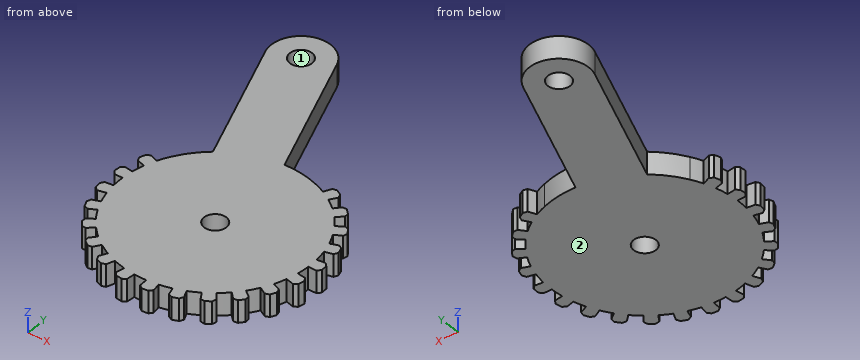
from build123d import *

# Parameters (mm, degrees)
SKETCH1_R           = 1.5
BOSS_EXTRUDE2_DEPTH = 3


with BuildPart() as part:
    # Sketch1 → Boss-Extrude2 (new body)
    with BuildSketch(Plane.XY):
        with BuildLine():
            Line((-15.222508379, 27.299729644), (-8.208462227, 9.756210733))
            ThreePointArc((-8.208462227, 9.756210733), (-9.850646229, 8.094891529), (-11.162172719, 6.161850387))
            ThreePointArc((-11.162172719, 6.161850387), (-11.536544919, 5.428685967), (-11.862823992, 4.672890641))
            Line((-11.862823992, 4.672890641), (-12.909543756, 5.085204521))
            Line((-12.909543756, 5.085204521), (-13.417390562, 4.799596912))
            Line((-13.417390562, 4.799596912), (-13.676029266, 4.003588828))
            Line((-13.676029266, 4.003588828), (-13.43304851, 3.474022556))
            Line((-13.43304851, 3.474022556), (-12.343882415, 3.192345052))
            ThreePointArc((-12.343882415, 3.192345052), (-12.524162447, 2.389111761), (-12.652232208, 1.575918828))
            Line((-12.652232208, 1.575918828), (-13.768605638, 1.71497049))
            Line((-13.768605638, 1.71497049), (-14.189469779, 1.312039404))
            Line((-14.189469779, 1.312039404), (-14.242023712, 0.476718548))
            Line((-14.242023712, 0.476718548), (-13.874978867, 0.024216431))
            Line((-13.874978867, 0.024216431), (-12.749980581, 0.022252937))
            ThreePointArc((-12.749980581, 0.022252937), (-12.724840787, -0.800579124), (-12.646654143, -1.62007376))
            Line((-12.646654143, -1.62007376), (-13.762535391, -1.763021444))
            Line((-13.762535391, -1.763021444), (-14.069972424, -2.257958364))
            Line((-14.069972424, -2.257958364), (-13.91313943, -3.080105712))
            Line((-13.91313943, -3.080105712), (-13.445093273, -3.427111302))
            Line((-13.445093273, -3.427111302), (-12.354950575, -3.149237412))
            ThreePointArc((-12.354950575, -3.149237412), (-12.125970583, -3.939966678), (-11.846440287, -4.714271155))
            Line((-11.846440287, -4.714271155), (-12.89171443, -5.130236257))
            Line((-12.89171443, -5.130236257), (-13.066406957, -5.686080305))
            Line((-13.066406957, -5.686080305), (-12.710041429, -6.443395602))
            Line((-12.710041429, -6.443395602), (-12.170403021, -6.663101027))
            Line((-12.170403021, -6.663101027), (-11.183613587, -6.122849592))
            ThreePointArc((-11.183613587, -6.122849592), (-10.76518105, -6.831791636), (-10.30187102, -7.512253556))
            Line((-10.30187102, -7.512253556), (-11.210859639, -8.175099458))
            Line((-11.210859639, -8.175099458), (-11.241831085, -8.756924908))
            Line((-11.241831085, -8.756924908), (-10.70832478, -9.401823249))
            Line((-10.70832478, -9.401823249), (-10.131001588, -9.48042361))
            Line((-10.131001588, -9.48042361), (-9.309569027, -8.711740614))
            ThreePointArc((-9.309569027, -8.711740614), (-8.727975601, -9.29435), (-8.109997309, -9.838213438))
            Line((-8.109997309, -9.838213438), (-8.825585306, -10.706291095))
            Line((-8.825585306, -10.706291095), (-8.710889622, -11.277539713))
            Line((-8.710889622, -11.277539713), (-8.033764703, -11.769499764))
            Line((-8.033764703, -11.769499764), (-7.455032066, -11.702056311))
            Line((-7.455032066, -11.702056311), (-6.850570006, -10.753240934))
            ThreePointArc((-6.850570006, -10.753240934), (-6.142359345, -11.172910171), (-5.40854264, -11.546002187))
            Line((-5.40854264, -11.546002187), (-5.885766991, -12.564767086))
            Line((-5.885766991, -12.564767086), (-5.632610928, -13.089545223))
            Line((-5.632610928, -13.089545223), (-4.854413643, -13.397655324))
            Line((-4.854413643, -13.397655324), (-4.310635461, -13.188405776))
            Line((-4.310635461, -13.188405776), (-3.961124478, -12.119075578))
            ThreePointArc((-3.961124478, -12.119075578), (-3.170796061, -12.349435304), (-2.367249346, -12.528313156))
            Line((-2.367249346, -12.528313156), (-2.576124288, -13.633752552))
            Line((-2.576124288, -13.633752552), (-2.200414573, -14.079086466))
            Line((-2.200414573, -14.079086466), (-1.370041921, -14.183986927))
            Line((-1.370041921, -14.183986927), (-0.895385777, -13.846079204))
            Line((-0.895385777, -13.846079204), (-0.82278693, -12.723424133))
            ThreePointArc((-0.82278693, -12.723424133), (0, -12.75), (0.82278693, -12.723424133))
            Line((0.82278693, -12.723424133), (0.895385777, -13.846079204))
            Line((0.895385777, -13.846079204), (1.370041921, -14.183986927))
            Line((1.370041921, -14.183986927), (2.200414573, -14.079086466))
            Line((2.200414573, -14.079086466), (2.576124288, -13.633752552))
            Line((2.576124288, -13.633752552), (2.367249346, -12.528313156))
            ThreePointArc((2.367249346, -12.528313156), (3.170796061, -12.349435304), (3.961124478, -12.119075578))
            Line((3.961124478, -12.119075578), (4.310635461, -13.188405776))
            Line((4.310635461, -13.188405776), (4.854413643, -13.397655324))
            Line((4.854413643, -13.397655324), (5.632610928, -13.089545223))
            Line((5.632610928, -13.089545223), (5.885766991, -12.564767086))
            Line((5.885766991, -12.564767086), (5.40854264, -11.546002187))
            ThreePointArc((5.40854264, -11.546002187), (6.142359345, -11.172910171), (6.850570006, -10.753240934))
            Line((6.850570006, -10.753240934), (7.455032066, -11.702056311))
            Line((7.455032066, -11.702056311), (8.033764703, -11.769499764))
            Line((8.033764703, -11.769499764), (8.710889622, -11.277539713))
            Line((8.710889622, -11.277539713), (8.825585306, -10.706291095))
            Line((8.825585306, -10.706291095), (8.109997309, -9.838213438))
            ThreePointArc((8.109997309, -9.838213438), (8.727975601, -9.29435), (9.309569027, -8.711740614))
            Line((9.309569027, -8.711740614), (10.131001588, -9.48042361))
            Line((10.131001588, -9.48042361), (10.70832478, -9.401823249))
            Line((10.70832478, -9.401823249), (11.241831085, -8.756924908))
            Line((11.241831085, -8.756924908), (11.210859639, -8.175099458))
            Line((11.210859639, -8.175099458), (10.30187102, -7.512253556))
            ThreePointArc((10.30187102, -7.512253556), (10.76518105, -6.831791636), (11.183613587, -6.122849592))
            Line((11.183613587, -6.122849592), (12.170403021, -6.663101027))
            Line((12.170403021, -6.663101027), (12.710041429, -6.443395602))
            Line((12.710041429, -6.443395602), (13.066406957, -5.686080305))
            Line((13.066406957, -5.686080305), (12.89171443, -5.130236257))
            Line((12.89171443, -5.130236257), (11.846440287, -4.714271155))
            ThreePointArc((11.846440287, -4.714271155), (12.125970583, -3.939966678), (12.354950575, -3.149237412))
            Line((12.354950575, -3.149237412), (13.445093273, -3.427111302))
            Line((13.445093273, -3.427111302), (13.91313943, -3.080105712))
            Line((13.91313943, -3.080105712), (14.069972424, -2.257958364))
            Line((14.069972424, -2.257958364), (13.762535391, -1.763021444))
            Line((13.762535391, -1.763021444), (12.646654143, -1.62007376))
            ThreePointArc((12.646654143, -1.62007376), (12.724840787, -0.800579124), (12.749980581, 0.022252937))
            Line((12.749980581, 0.022252937), (13.874978867, 0.024216431))
            Line((13.874978867, 0.024216431), (14.242023712, 0.476718548))
            Line((14.242023712, 0.476718548), (14.189469779, 1.312039404))
            Line((14.189469779, 1.312039404), (13.768605638, 1.71497049))
            Line((13.768605638, 1.71497049), (12.652232208, 1.575918828))
            ThreePointArc((12.652232208, 1.575918828), (12.524162447, 2.389111761), (12.343882415, 3.192345052))
            Line((12.343882415, 3.192345052), (13.43304851, 3.474022556))
            Line((13.43304851, 3.474022556), (13.676029266, 4.003588828))
            Line((13.676029266, 4.003588828), (13.417390562, 4.799596912))
            Line((13.417390562, 4.799596912), (12.909543756, 5.085204521))
            Line((12.909543756, 5.085204521), (11.862823992, 4.672890641))
            ThreePointArc((11.862823992, 4.672890641), (11.536544919, 5.428685967), (11.162172719, 6.161850387))
            Line((11.162172719, 6.161850387), (12.147070312, 6.705543068))
            Line((12.147070312, 6.705543068), (12.250719604, 7.278898898))
            Line((12.250719604, 7.278898898), (11.80224735, 7.985578094))
            Line((11.80224735, 7.985578094), (11.239327761, 8.13591645))
            Line((11.239327761, 8.13591645), (10.328030916, 7.476247548))
            ThreePointArc((10.328030916, 7.476247548), (9.824043845, 8.127155869), (9.27910266, 8.744184))
            Line((9.27910266, 8.744184), (10.097847012, 9.515729647))
            Line((10.097847012, 9.515729647), (10.055652175, 10.096848981))
            Line((10.055652175, 10.096848981), (9.445525531, 10.669796035))
            Line((9.445525531, 10.669796035), (8.862903468, 10.675418826))
            Line((8.862903468, 10.675418826), (8.144289673, 9.809844327))
            ThreePointArc((8.144289673, 9.809844327), (7.494261967, 10.314966678), (6.812992455, 10.777088374))
            Line((6.812992455, 10.777088374), (7.414138848, 11.728007936))
            Line((7.414138848, 11.728007936), (7.228751137, 12.280376908))
            Line((7.228751137, 12.280376908), (6.495306606, 12.683591451))
            Line((6.495306606, 12.683591451), (5.929590354, 12.544145377))
            Line((5.929590354, 12.544145377), (5.448812758, 11.527052508))
            ThreePointArc((5.448812758, 11.527052508), (4.733275563, 11.838859846), (4, 12.106300013))
            ThreePointArc((4, 12.106300013), (1.639477491, 12.644153335), (-0.78015801, 12.726109126))
            Line((-0.78015801, 12.726109126), (-7.794204162, 30.269628037))
            ThreePointArc((-7.794204162, 30.269628037), (-12.993305466, 32.498830949), (-15.222508379, 27.299729644))
        make_face()
        Circle(SKETCH1_R, mode=Mode.SUBTRACT)
        with Locations((-11.50835627, 28.784678841)):
            Circle(SKETCH1_R, mode=Mode.SUBTRACT)
    extrude(amount=BOSS_EXTRUDE2_DEPTH)


solid = part.part
For this review, take the finished solid that the model builds, in its own axes (mm). Face numbers are marked on the shaded views. Round coordinates to 2 decimals unless told otherwise and drop trailing zeros. Order: outer loops, then holes, each group sorted by start corner. A loop starts at its lowest first (then second) coordinate and runs counter-clockwise, first axis right, second up. Notation, with made-up numbers: (25.25, 57) -> (83.25, 57) arc R22 cw to (83.25, 86) -> close; hole circle Ø7 at (72, 28). An arc over 180 degrees is marked (long way). Write item = value, one per line. Start each with the question number.
1) To check wall thickness, follow line 1 (Y direction, x = 7, z = 2.75); line 2 (Y direction, x = 1, z = 2.55); line 3 (X direction, y = -6, z = 1.25). State the ranges of each line that lie inside material, in increasing order. Write a range as from..to.
2) Take a section at A-A on x = 0. State the section outline as (y, z) points, plus the area to 3 significant figures.
3) Take a section at C-C on z = 2. Count the separate pieces of the cut face and the enclosed holes in it, plus the area to 3 significant figures.
4) The part is to be moulded in two halves that separate along Y. For the marked faces 1 and 2, say which applies: +Y half, -Y half, draft (parallel to the pull), parting line (faces both ways), or undercut.
5) Take a section at B-B on y = 28. State the section outline as (x, z) points.
6) Insertion check: pin 1 (1 mm diameter, centred on x = 0.5, z = 2, fed in from +Y); pin 2 (1 mm diameter, centred on y = -5.5, z = 2, fed in from +X). Each pin has a flat end and moves straight along its axis. Give the tip position at first contact, or say it passes through.
Verdict:
q1.line_1 = -10.99..10.66, 11.07..12.41
q1.line_2 = -13.92..-1.12, 1.12..12.71
q1.line_3 = -12.92..12.92
q2.outline = (-12.75, 0) -> (-1.5, 0) -> (-1.5, 3) -> (-12.75, 3) -> close; (1.5, 0) -> (12.75, 0) -> (12.75, 3) -> (1.5, 3) -> close
q2.area = 67.5 mm2
q3.separate_pieces = 1
q3.enclosed_holes = 2
q3.area = 713 mm2
q4.face_1 = undercut
q4.face_2 = draft
q5.outline = (-15.43, 0) -> (-12.79, 0) -> (-12.79, 3) -> (-15.43, 3) -> close; (-10.23, 0) -> (-6.89, 0) -> (-6.89, 3) -> (-10.23, 3) -> close
q6.pin_1 = 12.75
q6.pin_2 = 13.07
